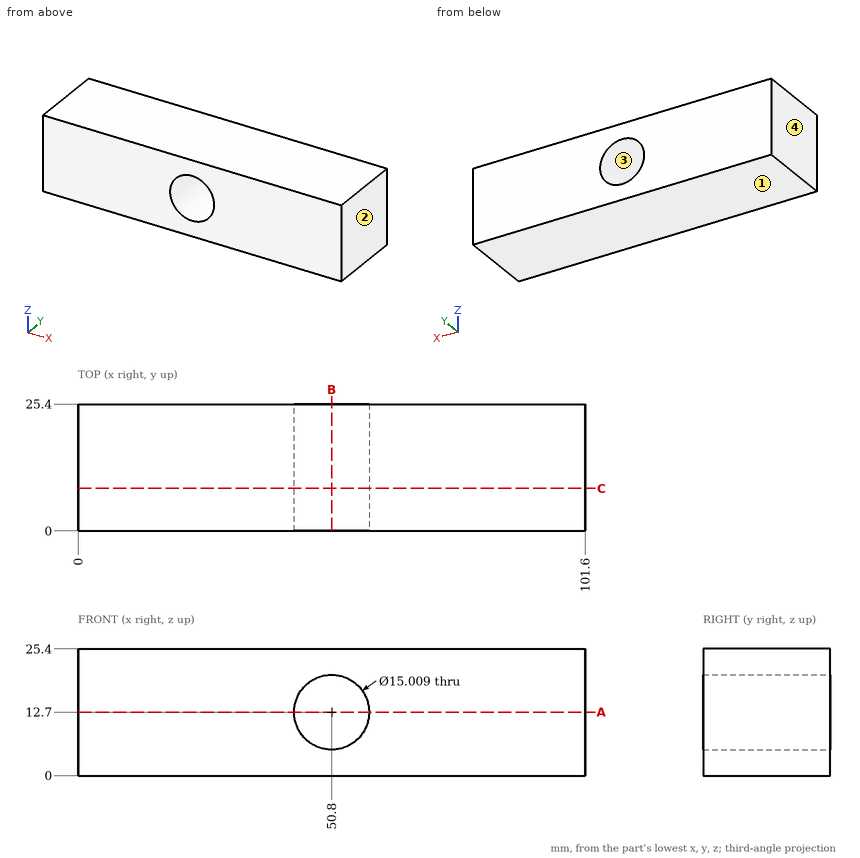
Job drawing, mm, ordinate dimensions from the low corner. One solid piece. Give positions to 0.01 mm unless a question says otherwise; leave off trailing zeros. Loops run counter-clockwise (first coordinate to the right, second up) from the corner with the lowest first, then second, coordinate; pieces in that order, holes last. Notation, with made-up numbers: (28.5, -10) - (54.5, -10) arc R15 cw to (54.5, -3) - close; hole circle Ø5 at (3.25, 40.5). An arc over 180 degrees is marked (long way). Use one line per item in the form item = value.
(1) Cut at A-A (z = 12.7). Give the cut face in (x, y) (1 decimal), then the cut area to 3 significant figures.
Determined:
outline = (0, 0) - (43.3, 0) - (43.3, 25.4) - (0, 25.4) - close; (58.3, 0) - (101.6, 0) - (101.6, 25.4) - (58.3, 25.4) - close
area = 2,200 mm^2
(2) Pull direction X, two halves, no side cores. Call the marked faces 1, 2, 3 and 4: pulls with the +X half, pulls with the -X half, needs draft (parallel to the pull), parting line crosses it, or undercut.
Determined:
face_1 = needs draft
face_2 = pulls with the +X half
face_3 = undercut
face_4 = pulls with the -X half
(3) Cut at B-B (x = 50.8). Give the cut face in (y, z) (1 decimal), then the cut area to 3 significant figures.
Determined:
outline = (0, 0) - (25.4, 0) - (25.4, 5.2) - (0, 5.2) - close; (0, 20.2) - (25.4, 20.2) - (25.4, 25.4) - (0, 25.4) - close
area = 264 mm^2
(4) Drill centre lines: L1, parallel to Z at x = 50.8, y = 18.5 (1 decimal); L2, parallel to X at y = 20.25, z = 16; L3, parallel to X at y = 4.5, z = 17. Where is each one in solid material? Low to high.
Determined:
L1 = 0 to 5.2, 20.2 to 25.4
L2 = 0 to 44.06, 57.54 to 101.6
L3 = 0 to 44.65, 56.95 to 101.6
(5) Cut at C-C (y = 8.5). Give the cut face in (x, z) (1 decimal).
Determined:
outline = (0, 0) - (101.6, 0) - (101.6, 25.4) - (0, 25.4) - close; hole circle Ø15 at (50.8, 12.7)
